Geometry: see drawing. Coordinates: mm, zero at the bounding-box minimum. Coordinates: 2 decimals unless noted, no trailing zeros. Loops run counter-clockwise (first coordinate to the right, second up) from the corner with the lowest first, then second, coordinate; pieces in that order, holes last. Notation, with made-up numbers: M 83,33.5 L 110,33.5 A19 cw 110,40.5 Z; hole C -21,-22.5 d6. An arc over 180 degrees is marked long. One line per question, with ' | ' between items. Start each with the question number.
1. Section query A-A, the plane y = 53.82. Output: boundary loops of the cut face in (x, z), and give its area (3 significant figures).
2. Mould query, pull axis Y, two halves, no side actions, for the marked faces 1, 2 and 3. Classes: pulls with the +Y half, pulls with the -Y half, needs draft (parallel to the pull), parting line crosses it, or undercut.
3. Section query D-D, the plane y = 30.25. Output: boundary loops of the cut face in (x, z).
4. Section query B-B, the plane x = 75. Output: boundary loops of the cut face in (y, z).
5. Pin query (flat end, axial travel): P1, Ø4, axis at x = 16.43, y = 6.68, coming from the +Z side. Return the tip coordinate at first contact, or that it passes through.
6. Section query C-C, the plane z = 8.5. Output: boundary loops of the cut face in (x, y).
7. Ray query, probe 1 along Y at (x, z) = (16.43, 3.75); probe 2 along X at (y, z) = (5.5, 8.25); probe 3 along Y at (x, z) = (18.5, 4). Return the intervals inside material, ascending.
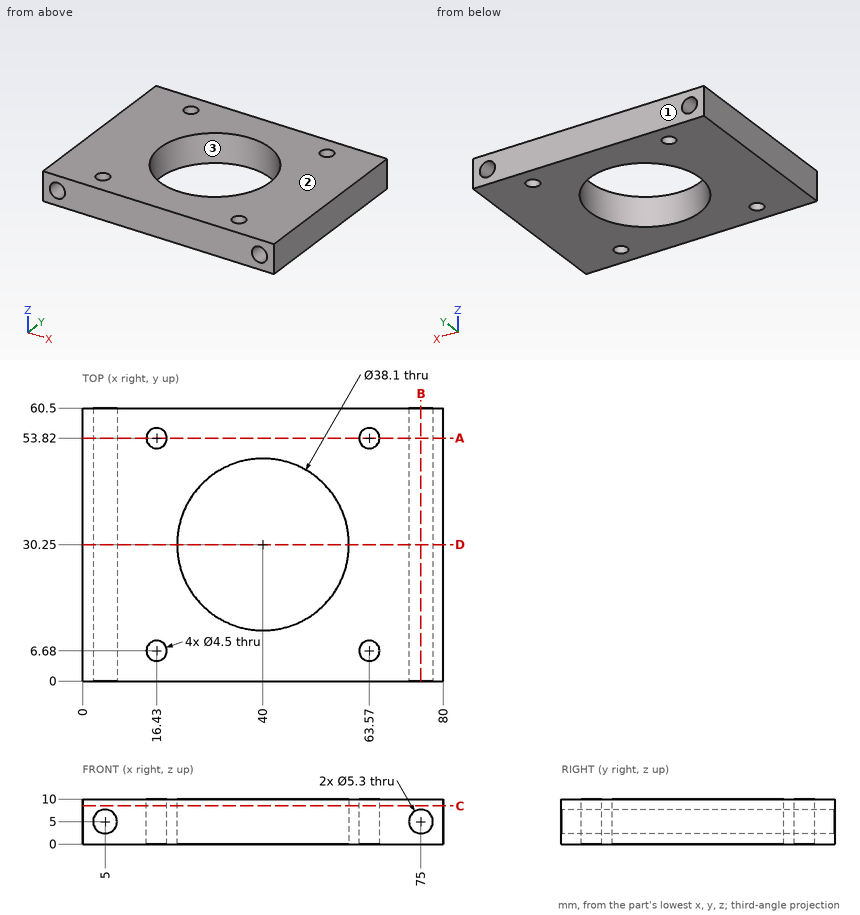
Taken from the geometry:
1) outline: M 0,0 L 14.18,0 L 14.18,10 L 0,10 Z; M 18.68,0 L 61.32,0 L 61.32,10 L 18.68,10 Z; M 65.82,0 L 80,0 L 80,10 L 65.82,10 Z; hole C 5,5 d5.3; hole C 75,5 d5.3 | area: 666 mm^2
2) face 1: pulls with the +Y half | face 2: needs draft | face 3: undercut
3) outline: M 0,0 L 20.95,0 L 20.95,10 L 0,10 Z; M 59.05,0 L 80,0 L 80,10 L 59.05,10 Z; hole C 5,5 d5.3; hole C 75,5 d5.3
4) outline: M 0,0 L 60.5,0 L 60.5,2.35 L 0,2.35 Z; M 0,7.65 L 60.5,7.65 L 60.5,10 L 0,10 Z
5) P1: through
6) outline: M 0,0 L 80,0 L 80,60.5 L 0,60.5 Z; hole C 16.43,6.68 d4.5; hole C 16.43,53.82 d4.5; hole C 40,30.25 d38.1; hole C 63.57,6.68 d4.5; hole C 63.57,53.82 d4.5
7) probe 1: 0 to 4.43, 8.93 to 51.57, 56.07 to 60.5 | probe 2: 0 to 14.51, 18.35 to 61.65, 65.49 to 80 | probe 3: 0 to 5.8, 7.56 to 52.94, 54.7 to 60.5
